Geometry: final body of the model. Coordinates: model frame, mm. Face numbers are marked on the shaded views. A direction names the side the tool comes from. Give positions to 0.01 mm unless a question says otherwise; leave off trailing zeros. Write each loop counter-clockwise with the first axis right and the second up, starting at its lowest first coordinate (ties: lowest second). Pieces come first, ordered by that corner, then holes. Notation, with made-up numbers: (62.25, -14.5) - (94.25, -14.5) arc R13 cw to (94.25, 9.5) - close; hole circle Ø4 at (-24, 89.5). An arc over 180 degrees is marked (long way). Return JSON: item names as keys, results as strings.
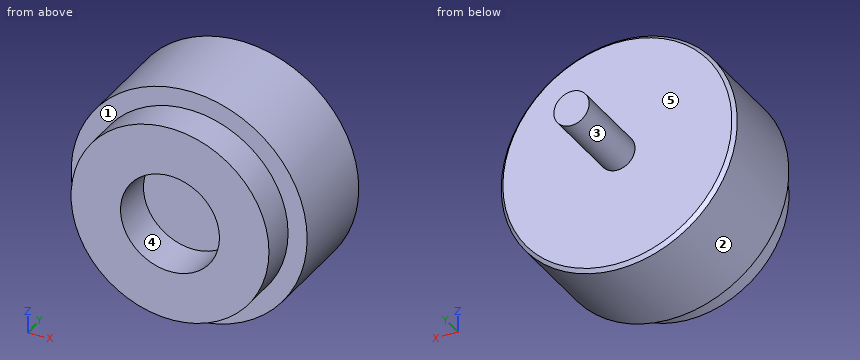
from build123d import *

# Parameters (mm, degrees)
SKETCH1_R           = 14
BOSS_EXTRUDE1_DEPTH = 5
SKETCH2_R           = 16.7
BOSS_EXTRUDE2_DEPTH = 14
SKETCH3_R           = 2.5
BOSS_EXTRUDE3_DEPTH = 12
CHAMFER1_SIZE       = 0.5
SKETCH4_R           = 7
CUT_EXTRUDE1_DEPTH  = 6


with BuildPart() as part:
    # Sketch1 → Boss-Extrude1 (new body)
    with BuildSketch(Plane(origin=(0, 0, 0), x_dir=(1, 0, 0), z_dir=(0, 1, 0))):
        Circle(SKETCH1_R)
    extrude(amount=BOSS_EXTRUDE1_DEPTH)

    # Sketch2 → Boss-Extrude2 (add)
    with BuildSketch(Plane(origin=(0, 5, 0), x_dir=(1, 0, 0), z_dir=(0, 1, 0))):
        Circle(SKETCH2_R)
    extrude(amount=BOSS_EXTRUDE2_DEPTH)

    # Sketch3 → Boss-Extrude3 (add)
    with BuildSketch(Plane(origin=(0, 19, 0), x_dir=(1, 0, 0), z_dir=(0, 1, 0))):
        Circle(SKETCH3_R)
    extrude(amount=BOSS_EXTRUDE3_DEPTH)

    # Chamfer1
    chamfer1_edges = [part.edges().sort_by_distance(p)[0] for p in [
        (-16.7, 19, 0),
    ]]
    chamfer(chamfer1_edges, length=CHAMFER1_SIZE)

    # Sketch4 → Cut-Extrude1 (cut)
    with BuildSketch(Plane.XZ):
        Circle(SKETCH4_R)
    extrude(amount=-CUT_EXTRUDE1_DEPTH, mode=Mode.SUBTRACT)


solid = part.part
Q1. Mould query, pull axis Z, two halves, no side actions, for the marked faces 3, 4 and 5. Classes: pulls with the +Z half, pulls with the -Z half, needs draft (parallel to the pull), parting line crosses it, or undercut.
Answer key:
{"face 3": "parting line crosses it", "face 4": "undercut", "face 5": "needs draft"}
Q2. Pin query (flat end, axial travel): P1, Ø2, axis at y = 12.5, z = 5.5, coming from the -X side; P2, Ø8, axis at y = 22.5, z = 9.5, coming from the -X side; P3, Ø2, axis at x = 6, y = 5.5, coming from the +Z side. Return the tip coordinate at first contact, or that it passes through.
Answer key:
{"P1": "stops at x = -16.08", "P2": "stops at x = -14.34", "P3": "stops at z = 15.93"}
Q3. Section query B-B, the plane z = 0. Return the cut outline in (x, y).
Answer key:
{"outline": "(-16.7, 5) - (-14, 5) - (-14, 0) - (-7, 0) - (-7, 6) - (7, 6) - (7, 0) - (14, 0) - (14, 5) - (16.7, 5) - (16.7, 18.5) - (16.2, 19) - (2.5, 19) - (2.5, 31) - (-2.5, 31) - (-2.5, 19) - (-16.2, 19) - (-16.7, 18.5) - close"}
Q4. Section query D-D, the plane y = 9.5. Return the cut outline in (x, z), plus the area to 3 significant figures.
Answer key:
{"outline": "circle Ø33.4 at (0, 0)", "area": "876 mm^2"}
Q5. Set-up query: the marked faces 1 and 2. Return all of +Z, -Z, +X, -X, +Y, -Y with unobstructed straight access to the full face (end or side cutting, diameter ignored); none if empty.
Answer key:
{"face 1": "-Y", "face 2": "+Y, -Y"}
Q6. Material intervals for probe 1 along Z at (x, y) = (0, 2); probe 2 along Y at (x, z) = (2.5, 6.5); probe 3 along Y at (x, z) = (-9.5, -12), sorted ascending. Write a range as [from, to].
Answer key:
{"probe 1": "z = [-14, -7], [7, 14]", "probe 2": "y = [6, 19]", "probe 3": "y = [5, 19]"}
Q7. Section query A-A, the plane x = 0. Return the cut outline in (y, z).
Answer key:
{"outline": "(0, -14) - (5, -14) - (5, -16.7) - (18.5, -16.7) - (19, -16.2) - (19, -2.5) - (31, -2.5) - (31, 2.5) - (19, 2.5) - (19, 16.2) - (18.5, 16.7) - (5, 16.7) - (5, 14) - (0, 14) - (0, 7) - (6, 7) - (6, -7) - (0, -7) - close"}
Q8. Section query C-C, the plane y = 25. Return the cut outline in (x, z).
Answer key:
{"outline": "circle Ø5 at (0, 0)"}
